Verification items for the finished model (mm, model axes). A direction names the side the tool comes from. Round coordinates to 2 decimals unless told otherwise and drop trailing zeros. Loops run counter-clockwise (first coordinate to the right, second up) from the corner with the lowest first, then second, coordinate; pieces in that order, holes last. Notation, with made-up numbers: (71.25, 43.25) -> (130.25, 43.25) arc R18 ccw to (130.25, 60.25) -> close; hole circle Ø10 at (-7, 40.25). An arc over 180 degrees is marked (long way). Write item = value, one per line.
```python
from build123d import *

# Parameters (mm, degrees)
SKETCH1_R             = 10
SKETCH1_R_2           = 1.5
SKETCH1_R_3           = 0.5
BOSS_EXTRUDE1_DEPTH   = 2
M3X0_5_TAPPED_HOLE2_D = 2.5
M3X0_5_TAPPED_HOLE3_D = 2.5
M3X0_5_TAPPED_HOLE4_D = 2.5
M3X0_5_TAPPED_HOLE5_D = 2.5
SKETCH11_R            = 4.5
SKETCH11_R_2          = 3.025
BOSS_EXTRUDE2_DEPTH   = 2.5


with BuildPart() as part:
    # Sketch1 → Boss-Extrude1 (new body)
    with BuildSketch(Plane.XY):
        Circle(SKETCH1_R)
        Circle(SKETCH1_R_2, mode=Mode.SUBTRACT)
        with Locations((-7, 0)):
            Circle(SKETCH1_R_3, mode=Mode.SUBTRACT)
        with Locations((0, 7)):
            Circle(SKETCH1_R_3, mode=Mode.SUBTRACT)
        with Locations((7, 0)):
            Circle(SKETCH1_R_3, mode=Mode.SUBTRACT)
        with Locations((0, -7)):
            Circle(SKETCH1_R_3, mode=Mode.SUBTRACT)
    extrude(amount=BOSS_EXTRUDE1_DEPTH)

    # M3x0.5 Tapped Hole2 (through all)
    with Locations(Plane(origin=(0, 7, 2), x_dir=(1, 0, 0), z_dir=(0, 0, 1))):
        with Locations((0, 0)):
            Hole(M3X0_5_TAPPED_HOLE2_D / 2)

    # M3x0.5 Tapped Hole3 (through all)
    with Locations(Plane.XY.offset(2)):
        with Locations((-7, 0)):
            Hole(M3X0_5_TAPPED_HOLE3_D / 2)

    # M3x0.5 Tapped Hole4 (through all)
    with Locations(Plane.XY.offset(2)):
        with Locations((0, -7)):
            Hole(M3X0_5_TAPPED_HOLE4_D / 2)

    # M3x0.5 Tapped Hole5 (through all)
    with Locations(Plane.XY.offset(2)):
        with Locations((7, 0)):
            Hole(M3X0_5_TAPPED_HOLE5_D / 2)

    # Sketch11 → Boss-Extrude2 (add)
    with BuildSketch(Plane.XY.offset(2)):
        Circle(SKETCH11_R)
        Circle(SKETCH11_R_2, mode=Mode.SUBTRACT)
    extrude(amount=BOSS_EXTRUDE2_DEPTH)


solid = part.part
```
(1) Sectioned sample at A-A, the plane y = 0. Record the cut outline in (x, z) (3 decimals).
Filled sheet:
outline = (-10, 0) -> (-8.25, 0) -> (-8.25, 2) -> (-10, 2) -> close; (-5.75, 0) -> (-1.5, 0) -> (-1.5, 2) -> (-3.025, 2) -> (-3.025, 4.5) -> (-4.5, 4.5) -> (-4.5, 2) -> (-5.75, 2) -> close; (1.5, 0) -> (5.75, 0) -> (5.75, 2) -> (4.5, 2) -> (4.5, 4.5) -> (3.025, 4.5) -> (3.025, 2) -> (1.5, 2) -> close; (8.25, 0) -> (10, 0) -> (10, 2) -> (8.25, 2) -> close
(2) Material ranges on probe 1 along Y at (x, z) = (0, 1.3); probe 2 along Y at (x, z) = (7, 1.8); probe 3 along Z at (x, y) = (-2.5, 6.5), recorded low to high. Write a range as from..to.
Filled sheet:
probe_1 = -10..-8.25, -5.75..-1.5, 1.5..5.75, 8.25..10
probe_2 = -7.14..-1.25, 1.25..7.14
probe_3 = 0..2
(3) Sectioned sample at D-D, the plane x = -7. Record the cut outline in (y, z), and give its area (3 significant figures).
Filled sheet:
outline = (-7.14, 0) -> (-1.25, 0) -> (-1.25, 2) -> (-7.14, 2) -> close; (1.25, 0) -> (7.14, 0) -> (7.14, 2) -> (1.25, 2) -> close
area = 23.6 mm2
(4) Set-up check for faces 5 (the face through (-0.59, 4.46, 3.23)), 6 (the face through (-1.5, 0.07, 0.99)): record each of +Z, -Z, +X, -X, +Y, -Y from which the full face is reachable in a straight line by a thin tool's end or side.
Filled sheet:
face_5 = +Z
face_6 = +Z, -Z
(5) Sectioned sample at B-B, the plane z = 1.15. Record the cut outline in (x, y), and give its area (3 significant figures).
Filled sheet:
outline = circle Ø20 at (0, 0); hole circle Ø2.5 at (-7, 0); hole circle Ø3 at (0, 0); hole circle Ø2.5 at (0, -7); hole circle Ø2.5 at (0, 7); hole circle Ø2.5 at (7, 0)
area = 287 mm2
(6) Go/stop test with flat-tipped pins: pin 1 Ø1.5 at (y, z) = (-1, 2) entering from +X; pin 2 Ø5 at (x, y) = (0, 0) entering from +Z. Record where each tip stops, or that it passes through.
Filled sheet:
pin_1 = 10
pin_2 = 2
(7) Draft check along Y on faces 1 (the face through (-2.17, -9.76, 0.99)), 2 (the face through (1.3, -1.3, 2)), 3 (the face through (4.3, -2.1, 2)), 4 (the face through (-5.75, 0.05, 0.99)). Enter one of: released by +Y, released by -Y, zero draft, split by the parting line, or undercut.
Filled sheet:
face_1 = split by the parting line
face_2 = undercut
face_3 = zero draft
face_4 = undercut
(8) Sectioned sample at C-C, the plane y = -6.5. Record the cut outline in (x, z), and give its area (3 significant figures).
Filled sheet:
outline = (-7.6, 0) -> (-1.15, 0) -> (-1.15, 2) -> (-7.6, 2) -> close; (1.15, 0) -> (7.6, 0) -> (7.6, 2) -> (1.15, 2) -> close
area = 25.8 mm2
